Geometry check sheet. Reference: the model listing, model coordinates, mm. Face numbers are marked on the shaded views. Coordinates: 2 decimals unless noted, no trailing zeros. Loops run counter-clockwise (first coordinate to the right, second up) from the corner with the lowest first, then second, coordinate; pieces in that order, holes last. Notation, with made-up numbers: (52.5, -18.75) - (94.5, -18.75) arc R23 ccw to (94.5, 18.25) - close; hole circle Ø6 at (26, 24). An arc over 180 degrees is marked (long way). One line per item, written item: value.
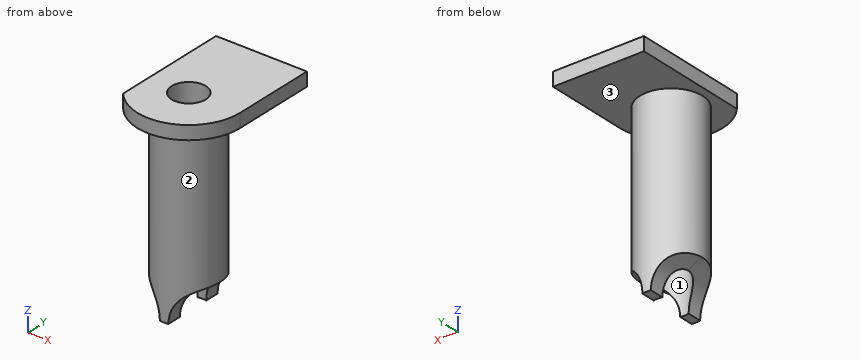
from build123d import *

# Parameters (mm, degrees)
F1_DEPTH      = 1.6
F2_R          = 3.65
F3_DEPTH      = 20.9
F4_R          = 4
F5_DEPTH      = 25
F5_DEPTH_BACK = 25
F6_R          = 2
F7_DEPTH      = 22.5010001


with BuildPart() as f1:
    # F0 (on Top) → F1 (new body)
    with BuildSketch(Plane.XY):
        with BuildLine():
            Line((-4.6, 9.8), (-4.6, -3.8522720569))
            ThreePointArc((-4.6, -3.8522720569), (2.0493901532, -5.6391488719), (6, 0))
            Line((6, 0), (6, 9.8))
            Line((6, 9.8), (-4.6, 9.8))
        make_face()
    extrude(amount=F1_DEPTH)

    # F2 (on face) → F3 (join)
    with BuildSketch(Plane(origin=(0, 0, 0), x_dir=(1, 0, 0), z_dir=(0, 0, -1))):
        Circle(F2_R)
    extrude(amount=F3_DEPTH)

    # F4 (on Front) → F5 (cut, two sides)
    with BuildSketch(Plane.XZ) as f5_sk:
        with Locations((4.5, -20.9)):
            Circle(F4_R)
        with Locations((-4.5, -20.9)):
            Circle(F4_R)
    extrude(amount=-F5_DEPTH, mode=Mode.SUBTRACT)
    extrude(f5_sk.sketch, amount=F5_DEPTH_BACK, mode=Mode.SUBTRACT)

    # F6 (on face) → F7 (cut, through all)
    with BuildSketch(Plane.XY.offset(1.6)):
        Circle(F6_R)
    extrude(amount=-F7_DEPTH, mode=Mode.SUBTRACT)


solid = f1.part
(1) Cross-section at C-C on z = -11.25. Record the cut outline in (x, y), and give its area (3 significant figures).
Reply:
outline: circle Ø7.3 at (0, 0); hole circle Ø4 at (0, 0)
area: 29.3 mm2
(2) Material ranges on probe 1 along X at (y, z) = (0, -9.5); probe 2 along Z at (x, y) = (-2.75, -2.75), recorded low to high. Write a range as from..to.
Reply:
probe 1: -3.65..-2, 2..3.65
probe 2: 0..1.6
(3) Cross-section at B-B on y = 0.75. Record the cut outline in (x, z).
Reply:
outline: (-4.6, 0) - (-3.57, 0) - (-3.57, -17.01) arc R4 cw to (-1.85, -17.9) - (-1.85, 1.6) - (-4.6, 1.6) - close; (1.85, -17.9) arc R4 cw to (3.57, -17.01) - (3.57, 0) - (6, 0) - (6, 1.6) - (1.85, 1.6) - close
(4) Go/stop test with flat-tipped pins: pin 1 Ø2 at (x, z) = (1, -7.5) entering from +Y; pin 2 Ø3 at (x, y) = (0.5, -4) entering from -Z; pin 3 Ø1.5 at (x, z) = (2, -18) entering from -Y. Record where each tip stops, or that it passes through.
Reply:
pin 1: y = 3.65
pin 2: z = -20.9
pin 3: y = -3.43
(5) Cross-section at D-D on x = -2.5. Record the cut outline in (y, z), and give its area (3 significant figures).
Reply:
outline: (-5.45, 0) - (-2.66, 0) - (-2.66, -17.44) - (2.66, -17.44) - (2.66, 0) - (9.8, 0) - (9.8, 1.6) - (-5.45, 1.6) - close
area: 117 mm2
(6) Release check for a two-part mould opening along X. For the marked faces 1, 2 and 3 record: pulls with the +X half, pulls with the -X half, needs draft (parallel to the pull), parting line crosses it, or undercut.
Reply:
face 1: undercut
face 2: parting line crosses it
face 3: needs draft
(7) Cross-section at A-A on x = 0. Record the cut outline in (y, z).
Reply:
outline: (-6, 0) - (-3.65, 0) - (-3.65, -20.9) - (-2, -20.9) - (-2, 1.6) - (-6, 1.6) - close; (2, -20.9) - (3.65, -20.9) - (3.65, 0) - (9.8, 0) - (9.8, 1.6) - (2, 1.6) - close
